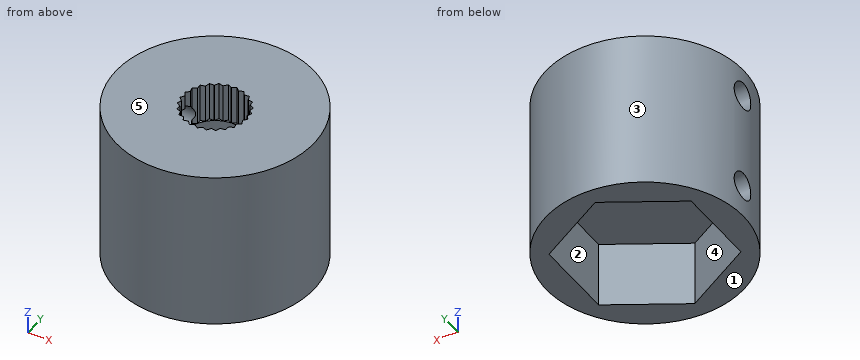
from build123d import *

# Parameters (mm, degrees)
SKETCH1_R           = 10
BOSS_EXTRUDE1_DEPTH = 2
SKETCH2_R           = 4.5
BOSS_EXTRUDE2_DEPTH = 2.5
SKETCH3_R           = 2.75
CUT_EXTRUDE1_DEPTH  = 5
CUT_EXTRUDE3_DEPTH  = 3.5
CIRPATTERN1_COUNT   = 25
SKETCH6_R           = 1.5
CUT_EXTRUDE4_DEPTH  = 15.361406616
FILLET1_R           = 0.1
THREAD1_PITCH       = 0.3175
CUT_EXTRUDE5_START  = -10
SKETCH7_R           = 11.568121222
SKETCH7_R_2         = 4.5
CUT_EXTRUDE5_DEPTH  = 10
BOSS_EXTRUDE3_START = 10
SKETCH8_R           = 4.5
BOSS_EXTRUDE3_DEPTH = 10
SKETCH9_R           = 9
SKETCH9_R_2         = 4.5
BOSS_EXTRUDE4_DEPTH = 14.5
CUT_EXTRUDE6_DEPTH  = 6
SKETCH11_R          = 1.25
CUT_EXTRUDE7_DEPTH  = 9


with BuildPart() as part:
    # Sketch1 → Boss-Extrude1 (new body)
    with BuildSketch(Plane.XY):
        Circle(SKETCH1_R)
    extrude(amount=BOSS_EXTRUDE1_DEPTH)

    # Sketch2 → Boss-Extrude2 (add)
    with BuildSketch(Plane.XY.offset(2)):
        Circle(SKETCH2_R)
    extrude(amount=BOSS_EXTRUDE2_DEPTH)

    # Sketch3 → Cut-Extrude1 (cut)
    with BuildSketch(Plane.XY.offset(4.5)):
        Circle(SKETCH3_R)
    extrude(amount=-CUT_EXTRUDE1_DEPTH, mode=Mode.SUBTRACT)

    # Sketch5 → Cut-Extrude3 (cut)
    with BuildSketch(Plane.XY.offset(4.5)):
        Polygon((-2.656507983, 0.682075321), (-2.682344512, 0.606240809), (-2.75, 0), (-2.976344104, 0.375999701), align=None)
    cut_extrude3 = extrude(amount=-CUT_EXTRUDE3_DEPTH, mode=Mode.SUBTRACT)

    # CirPattern1: Cut-Extrude3 ×25 about axis
    cirpattern1_axis = Axis((0, 0, 0), (0, 0, 1))
    for i in range(1, CIRPATTERN1_COUNT):
        add(cut_extrude3.rotate(cirpattern1_axis, i * 360 / CIRPATTERN1_COUNT), mode=Mode.SUBTRACT)

    # Sketch6 → Cut-Extrude4 (cut, through all)
    with BuildSketch(Plane.XY.offset(2)):
        with Locations((-7, 0)):
            Circle(SKETCH6_R)
        with Locations(Location((7, 0, 0), (0, 0, 180))):
            Circle(SKETCH6_R)
        with Locations(Location((0, 7, 0), (0, 0, 180))):
            Circle(SKETCH6_R)
        with Locations((0, -7)):
            Circle(SKETCH6_R)
    extrude(amount=-CUT_EXTRUDE4_DEPTH, mode=Mode.SUBTRACT)

    # Fillet1
    fillet1_edges = [part.edges().sort_by_distance(p)[0] for p in [
        (8.5, 0, 2),
    ]]
    fillet(fillet1_edges, radius=FILLET1_R)

    # Thread1: the profile of Thread Profile3 profile screwed along a right-hand helix of 6.299213 turns, 6 arcs to a turn; built about Z, then put on its axis
    thread1_z = Axis((0, 0, 0), (0, 0, 1))
    thread1_corners = [(1.5003, 0, -0.000173205), (1.5003, 0, 0.277985704), (1.328148085, 0, 0.17859375), (1.328148085, 0, 0.09921875)]
    with BuildLine(mode=Mode.PRIVATE) as thread1_profile:
        Line(thread1_corners[0], thread1_corners[1])
        Line(thread1_corners[1], thread1_corners[2])
        Line(thread1_corners[2], thread1_corners[3])
        Line(thread1_corners[3], thread1_corners[0])
    thread1_cap = Face(thread1_profile.wire())
    thread1_turn_angles = [0, 30, 60, 90, 120, 150, 180, 210, 240, 270, 300, 330, 360]
    thread1_turn_weights = [1, 0.8660254037844387, 1, 0.8660254037844387, 1, 0.8660254037844387, 1, 0.8660254037844387, 1, 0.8660254037844387, 1, 0.8660254037844387, 1]
    thread1_turn_rails = [Edge.make_bspline([Vector(p[0], p[1], 0).rotate(thread1_z, thread1_turn_angles[k]) / thread1_turn_weights[k] + Vector(0, 0, p[2] + THREAD1_PITCH * thread1_turn_angles[k] / 360) for k in range(13)], [0, 0, 0, 1, 1, 2, 2, 3, 3, 4, 4, 5, 5, 6, 6, 6], 2, thread1_turn_weights) for p in thread1_corners]
    thread1_turn_sides = [Face.make_surface_from_curves(thread1_turn_rails[p[0]], thread1_turn_rails[p[1]]) for p in [(0, 1), (1, 2), (2, 3), (3, 0)]]
    thread1_last_angles = [2160, 2190, 2220, 2243.858267717, 2267.716535433]
    thread1_last_weights = [1, 0.8660254037844387, 1, 0.9145488039507501, 1]
    thread1_last_rails = [Edge.make_bspline([Vector(p[0], p[1], 0).rotate(thread1_z, thread1_last_angles[k]) / thread1_last_weights[k] + Vector(0, 0, p[2] + THREAD1_PITCH * thread1_last_angles[k] / 360) for k in range(5)], [0, 0, 0, 1, 1, 2, 2, 2], 2, thread1_last_weights) for p in thread1_corners]
    thread1_last_sides = [Face.make_surface_from_curves(thread1_last_rails[p[0]], thread1_last_rails[p[1]]) for p in [(0, 1), (1, 2), (2, 3), (3, 0)]]
    thread1 = Plane(origin=(7, 0, 1.9), x_dir=(-1, 0, 0), z_dir=(0, 0, -1)) * Solid(Shell([*[p.moved(Location((0, 0, THREAD1_PITCH * i))) for i in range(6) for p in thread1_turn_sides], *thread1_last_sides, thread1_cap, thread1_cap.rotate(thread1_z, 2267.716535433).moved(Location((0, 0, THREAD1_PITCH * 2267.716535433 / 360)))]))
    add(thread1)

    # Sketch7 → Cut-Extrude5 (cut)
    with BuildSketch(Plane.XY.offset(4.5).offset(CUT_EXTRUDE5_START)):
        Circle(SKETCH7_R)
        Circle(SKETCH7_R_2, mode=Mode.SUBTRACT)
    extrude(amount=CUT_EXTRUDE5_DEPTH, mode=Mode.SUBTRACT)

    # Sketch8 → Boss-Extrude3 (add)
    with BuildSketch(Plane(origin=(0, 0, 0), x_dir=(-1, 0, 0), z_dir=(0, 0, -1)).offset(BOSS_EXTRUDE3_START)):
        Circle(SKETCH8_R)
    extrude(amount=-BOSS_EXTRUDE3_DEPTH)

    # Sketch9 → Boss-Extrude4 (add)
    # profile 1 of 2: a face of its own
    with BuildSketch(Plane(origin=(0, 0, -10), x_dir=(-1, 0, 0), z_dir=(0, 0, -1))):
        Circle(SKETCH9_R)
        Polygon((5, 2.886751346), (0, 5.773502692), (-5, 2.886751346), (-5, -2.886751346), (0, -5.773502692), (5, -2.886751346), align=None, mode=Mode.SUBTRACT)
    # profile 2 of 2: a face of its own
    with BuildSketch(Plane(origin=(0, 0, -10), x_dir=(-1, 0, 0), z_dir=(0, 0, -1))):
        Polygon((5, -2.886751346), (5, 2.886751346), (0, 5.773502692), (-5, 2.886751346), (-5, -2.886751346), (0, -5.773502692), align=None)
        Circle(SKETCH9_R_2, mode=Mode.SUBTRACT)
    extrude(amount=-BOSS_EXTRUDE4_DEPTH)

    # Sketch10 → Cut-Extrude6 (cut)
    with BuildSketch(Plane(origin=(0, 0, -10), x_dir=(-1, 0, 0), z_dir=(0, 0, -1))):
        Polygon((0, 7.505553499), (-6.5, 3.75277675), (-6.5, -3.75277675), (0, -7.505553499), (6.5, -3.75277675), (6.5, 3.75277675), align=None)
    extrude(amount=-CUT_EXTRUDE6_DEPTH, mode=Mode.SUBTRACT)

    # Sketch11 → Cut-Extrude7 (cut)
    with BuildSketch(Plane(origin=(0, 0, 0), x_dir=(0, 0, -1), z_dir=(1, 0, 0))):
        with Locations(Location((-1.940949094, 0, 0), (0, 0, 180.000000024))):
            Circle(SKETCH11_R)
        with Locations((7, 0)):
            Circle(SKETCH11_R)
    extrude(amount=-CUT_EXTRUDE7_DEPTH, mode=Mode.SUBTRACT)


solid = part.part
Read the model definition and answer for the solid it produces. Units are mm, in the model's axes. Face numbers are marked on the shaded views. A direction names the side the tool comes from. Give positions to 0.01 mm unless a question says otherwise; leave off trailing zeros. Write each loop counter-clockwise with the first axis right and the second up, starting at its lowest first coordinate (ties: lowest second). Pieces come first, ordered by that corner, then holes. Notation, with made-up numbers: (89.25, 62.25) - (120.25, 62.25) arc R13 cw to (120.25, 70.25) - close; hole circle Ø11 at (64, 11). An arc over 180 degrees is marked (long way). Use CSV: the item, a comma, the result in double quotes. Start each with the question number.
Item 1: The mould has two halves that part along X. Classify the marked faces 3, 4 and 5: pulls with the +X half, pulls with the -X half, needs draft (parallel to the pull), parting line crosses it, or undercut.
Item 2: The part is cut by section A-A, the plane z = -7. Give the vertices of the cut face in (x, y).
Item 3: The part is cut by section C-C, the plane y = 4. Give the vertices of the cut face in (x, z), and give its area (3 significant figures).
Item 4: The part is cut by section D-D, the plane z = -3.5. Give the vertices of the cut face in (x, y), and give its area (3 significant figures).
Item 5: For the marked faces 1 and 2, determine the directions among +Z, -Z, +X, -X, +Y, -Y from which every point of the face is accessible in a straight line to the end or side of a thin tool.
Item 6: Flat-ended cylindrical pins translate along their axes: P1, Ø10.5, axis at x = -0.5, y = 3.5, coming from the -Z side; P2, Ø2, axis at y = 6, z = 3, coming from the -X side; P3, Ø2, axis at y = 0, z = -7, coming from the -X side; P4, Ø8, axis at y = 6.5, z = -3, coming from the +X side. Find the tip coordinate at first contact, or state that the pin passes through.
Item 7: The part is cut by section B-B, the plane x = 4.5. Give the vertices of the cut face in (y, z).
Item 8: Consider line 1 (Z direction, x = 1.25, y = 5.5); line 2 (Y direction, x = -1.75, z = 2.5); line 3 (Y direction, x = 0, z = 1.55). Determine where each line is inside the solid, lowest interval first.
Taken from the geometry:
1,face 3,"parting line crosses it"
1,face 4,"undercut"
1,face 5,"needs draft"
2,outline,"(-8.91, -1.25) arc R9 ccw (long way) to (-8.91, 1.25) - (-6.5, 1.25) - (-6.5, 3.75) - (0, 7.51) - (6.5, 3.75) - (6.5, -3.75) - (0, -7.51) - (-6.5, -3.75) - (-6.5, -1.25) - close"
3,outline,"(-8.06, -10) - (-6.07, -10) - (-6.07, -4) - (6.07, -4) - (6.07, -10) - (8.06, -10) - (8.06, 4.5) - (-8.06, 4.5) - close"
3,area,"161 mm2"
4,outline,"circle Ø18 at (0, 0)"
4,area,"254 mm2"
5,face 1,"-Z, +X, -X, +Y, -Y"
5,face 2,"-Z"
6,P1,"z = -10"
6,P2,"x = -7.48"
6,P3,"x = 6.5"
6,P4,"x = 8.65"
7,outline,"(-7.79, -10) - (-4.91, -10) - (-4.91, -4) - (4.91, -4) - (4.91, -10) - (7.79, -10) - (7.79, 4.5) - (-7.79, 4.5) - close"
8,line 1,"-4 to 4.5"
8,line 2,"-8.83 to -2.32, 2.31 to 8.83"
8,line 3,"-9 to -2.86, 2.86 to 9"
